CAD build for the part. Positions are in the model's coordinates, mm. Face numbers are marked on the shaded views. Round coordinates to 2 decimals unless told otherwise and drop trailing zeros. Loops run counter-clockwise (first coordinate to the right, second up) from the corner with the lowest first, then second, coordinate; pieces in that order, holes last. Notation, with made-up numbers: M 33.5,-31.75 L 49.5,-31.75 A24 ccw 49.5,1.25 Z; hole C 47,49.25 d1. An arc over 180 degrees is marked long. Use a Markdown table: item, result. Add a question column.
(1) Band-saw the part on D-D, the plane y = 162. Write the cut outline in (x, z).
(2) Wall check: L1, parallel to Y at x = 30.5, z = 224.5; L2, parallel to Z at x = -253, y = 81; L3, parallel to Z at x = -200.5, y = 24.5. Give the ranges that are in metal, low to high.
(3) Two-plate mould, pull along Y, no slides. Class the marked faces 1, 2, 3 and 4: released by +Y, released by -Y, zero draft, split by the parting line, or undercut.
(4) Band-saw the part on A-A, the plane z = 0. Write the cut outline in (x, y).
(5) Flat gauge pins, fed straight in: P1, Ø2.5, axis at y = 72.5, z = 212, coming from the -X side; P2, Ø1.7, axis at y = 66.5, z = 211, coming from the +X side; P3, Ø4, axis at y = -187, z = 52, coming from the -X side. Where does each tip first touch, or does it go through?
(6) Band-saw the part on B-B, the plane x = 0. Write the cut outline in (y, z), and give its area (3 significant figures).
(7) Band-saw the part on C-C, the plane y = -354. Write the cut outline in (x, z), and give its area (3 significant figures).
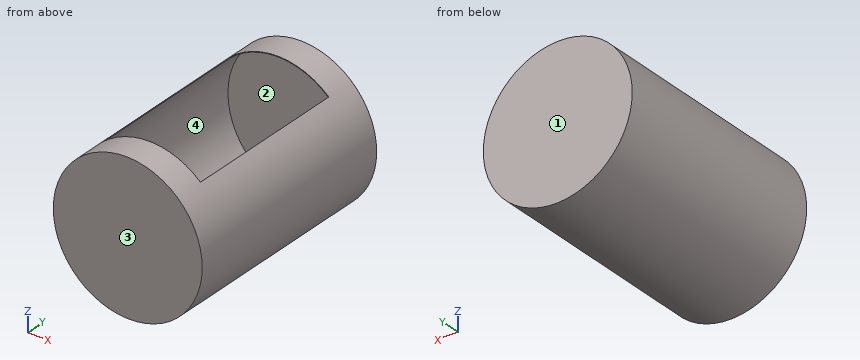
from build123d import *

# Parameters (mm, degrees)
F0_R     = 285.75
F1_DEPTH = 431.8
F2_W     = 381
F2_H     = 635
F3_DEPTH = 452.12
F4_T     = -2.54


with BuildPart() as f1:
    # F0 (on Front) → F1 (new body, symmetric)
    with BuildSketch(Plane.XZ):
        Circle(F0_R)
    extrude(amount=F1_DEPTH, both=True)

    # F2 (on Top) → F3 (cut)
    with BuildSketch(Plane.XY):
        Rectangle(F2_W, F2_H)
    extrude(amount=F3_DEPTH, mode=Mode.SUBTRACT)

    # F4
    f4_openings = [f1.faces().sort_by_distance(p)[0] for p in [
        (0, 317.5, 132.295443),
        (-190.5, 0, 106.492737),
        (0, 0, 0),
        (0, -317.5, 132.295443),
        (190.5, 0, 106.492737),
    ]]
    offset(amount=F4_T, openings=f4_openings)


solid = f1.part
Return value:
| question | item | result |
|---|---|---|
| 1 | outline | M -190.5,209.57 L -190.5,212.99 A285.75 ccw long 190.5,212.99 L 190.5,209.57 A283.21 cw long Z |
| 2 | L1 | -431.8 to -429.26, 429.26 to 431.8 |
| 2 | L2 | -132.83 to -127.27, 127.27 to 132.83 |
| 2 | L3 | -203.6 to -200.02, 200.02 to 203.6 |
| 3 | face 1 | released by +Y |
| 3 | face 2 | undercut |
| 3 | face 3 | released by -Y |
| 3 | face 4 | undercut |
| 4 | outline | M -285.75,-431.8 L 285.75,-431.8 L 285.75,431.8 L -285.75,431.8 Z; hole M -283.21,-429.26 L 283.21,-429.26 L 283.21,429.26 L -283.21,429.26 Z |
| 5 | P1 | x = -192.97 |
| 5 | P2 | x = 193.62 |
| 5 | P3 | x = -281.34 |
| 6 | outline | M -431.8,-285.75 L 431.8,-285.75 L 431.8,285.75 L 317.5,285.75 L 317.5,283.21 L 429.26,283.21 L 429.26,-283.21 L -429.26,-283.21 L -429.26,283.21 L -317.5,283.21 L -317.5,285.75 L -431.8,285.75 Z |
| 6 | area | 5,650 mm^2 |
| 7 | outline | C 0,0 d571.5; hole C 0,0 d566.42 |
| 7 | area | 4,540 mm^2 |
